Verification items for the finished model (mm, model axes). Coordinates: 2 decimals unless noted, no trailing zeros. Loops run counter-clockwise (first coordinate to the right, second up) from the corner with the lowest first, then second, coordinate; pieces in that order, holes last. Notation, with made-up numbers: (-13.75, 57) - (25.25, 57) arc R17 ccw to (25.25, 69) - close; hole circle Ø2 at (28.25, 78). An arc over 180 degrees is marked (long way). One line per item, written item: value. Start each with the question number.
(1) Section check B-B (z = -86). Count the separate pieces of the cut face and the enclosed holes in it, plus the area to 3 significant figures.
(2) Gauge pin test, flat ends, axial feed: P1, Ø20, axis at x = 83, z = -86, coming from the +Y side; P2, Ø6, axis at x = 338, z = -248, coming from the +Y side. Record the tip position at first contact, or that the pin passes through.
(3) Thickness scan on probe 1 along X at (y, z) = (-26, -86); probe 2 along X at (y, z) = (-2, -86); probe 3 along Z at (x, y) = (570.5, -4). Record the ranges inside material, lowest first. Write a range as [from, to].
(4) Section check A-A (x = 36). Record the boundary of the cut face in (y, z), plus the area to 3 significant figures.
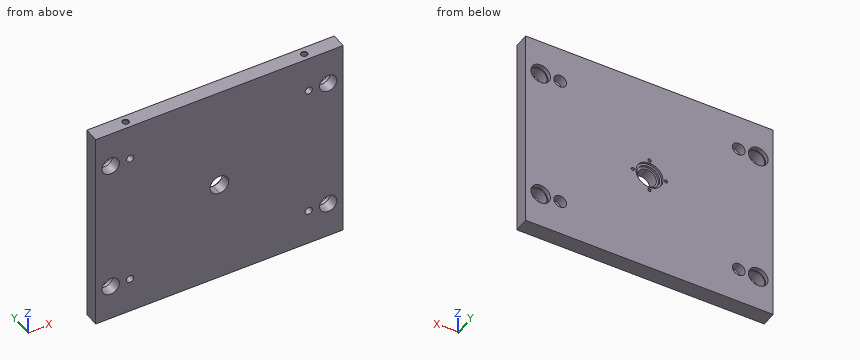
```python
from build123d import *

# Parameters (mm, degrees)
SZKIC1_W                                           = 596
SZKIC1_H                                           = 496
SZKIC1_R                                           = 45
SZKIC1_R_2                                         = 21
DODANIE_WYCI_GNI_CIE1_DEPTH                        = 36
POG_BIENIE_WALCOWE_POD_M16_WKR_T_Z_BEM_D           = 17.5
POG_BIENIE_WALCOWE_POD_M16_WKR_T_Z_BEM_CBORE_D     = 30.713
POG_BIENIE_WALCOWE_POD_M16_WKR_T_Z_BEM_CBORE_DEPTH = 21
SZKIC8_R                                           = 23.5
WYTNIJ_WYCI_GNI_CIE1_DEPTH                         = 10
WYTNIJ_WYCI_GNI_CIE3_DEPTH                         = 777.226770989
WYTNIJ_WYCI_GNI_CIE4_DEPTH                         = 10
WYTNIJ_WYCI_GNI_CIE5_DEPTH                         = 5
OTW_R_GWINTOWANY_M161_D                            = 14
OTW_R_GWINTOWANY_M161_DEPTH                        = 42
OTW_R_GWINTOWANY_M161_CSINK_D                      = 16.05
OTW_R_GWINTOWANY_M161_CSINK_ANGLE                  = 90
OTW_R_GWINTOWANY_M161_TIP                          = 4.206024333
OTW_R_GWINTOWANY_M81_D                             = 6.8
OTW_R_GWINTOWANY_M81_DEPTH                         = 22.25
OTW_R_GWINTOWANY_M81_CSINK_D                       = 8.05
OTW_R_GWINTOWANY_M81_CSINK_ANGLE                   = 90
OTW_R_GWINTOWANY_M81_TIP                           = 2.042926105


with BuildPart() as part:
    # Szkic1 → Dodanie-wyci_gni_cie1 (new body)
    # profile 1 of 2: a face of its own
    with BuildSketch(Plane(origin=(0, 0, 0), x_dir=(1, 0, 0), z_dir=(0, 1, 0))):
        with Locations((298, 248)):
            Rectangle(SZKIC1_W, SZKIC1_H)
        with Locations((298, 248)):
            Circle(SZKIC1_R, mode=Mode.SUBTRACT)
        with Locations(Location((560, 410, 0), (0, 0, 270))):
            Circle(SZKIC1_R_2, mode=Mode.SUBTRACT)
        with Locations(Location((36, 410, 0), (0, 0, 270))):
            Circle(SZKIC1_R_2, mode=Mode.SUBTRACT)
        with Locations(Location((560, 86, 0), (0, 0, 270))):
            Circle(SZKIC1_R_2, mode=Mode.SUBTRACT)
        with Locations(Location((36, 86, 0), (0, 0, 270))):
            Circle(SZKIC1_R_2, mode=Mode.SUBTRACT)
    # profile 2 of 2: a face of its own
    with BuildSketch(Plane(origin=(0, 0, 0), x_dir=(1, 0, 0), z_dir=(0, 1, 0))):
        with Locations((298, 248)):
            Circle(SZKIC1_R)
    extrude(amount=-DODANIE_WYCI_GNI_CIE1_DEPTH)

    # Pog_bienie walcowe pod M16 Wkr_t z _bem (through all)
    with Locations(Plane(origin=(83, 0, -410), x_dir=(0, 0, 1), z_dir=(0, 1, 0))):
        with Locations((0, 0), (0, 430), (324, 430), (324, 0)):
            CounterBoreHole(POG_BIENIE_WALCOWE_POD_M16_WKR_T_Z_BEM_D / 2, POG_BIENIE_WALCOWE_POD_M16_WKR_T_Z_BEM_CBORE_D / 2, POG_BIENIE_WALCOWE_POD_M16_WKR_T_Z_BEM_CBORE_DEPTH)

    # Szkic8 → Wytnij-wyci_gni_cie1 (cut)
    with BuildSketch(Plane(origin=(0, 0, 0), x_dir=(1, 0, 0), z_dir=(0, 1, 0))):
        with Locations(Location((36, 410, 0), (0, 0, 270))):
            Circle(SZKIC8_R)
        with Locations(Location((560, 410, 0), (0, 0, 90))):
            Circle(SZKIC8_R)
        with Locations(Location((560, 86, 0), (0, 0, 270))):
            Circle(SZKIC8_R)
        with Locations(Location((36, 86, 0), (0, 0, 90))):
            Circle(SZKIC8_R)
    extrude(amount=-WYTNIJ_WYCI_GNI_CIE1_DEPTH, mode=Mode.SUBTRACT)

    # Szkic10 → Wytnij-wyci_gni_cie3 (cut, through all)
    with BuildSketch(Plane(origin=(0, 0, 0), x_dir=(1, 0, 0), z_dir=(0, 1, 0))):
        with BuildLine():
            ThreePointArc((320.5, 248), (313.909902577, 263.909902577), (298, 270.5))
            Line((298, 270.5), (298, 225.5))
            ThreePointArc((298, 225.5), (313.909902577, 232.090097423), (320.5, 248))
        make_face()
        with BuildLine():
            Line((298, 225.5), (298, 270.5))
            ThreePointArc((298, 270.5), (275.5, 248), (298, 225.5))
        make_face()
    extrude(amount=-WYTNIJ_WYCI_GNI_CIE3_DEPTH, mode=Mode.SUBTRACT)

    # Szkic10_3 → Wytnij-wyci_gni_cie4 (cut)
    with BuildSketch(Plane(origin=(0, 0, 0), x_dir=(1, 0, 0), z_dir=(0, 1, 0))):
        with BuildLine():
            ThreePointArc((325.5, 248), (317.445436483, 267.445436483), (298, 275.5))
            Line((298, 275.5), (298, 270.5))
            ThreePointArc((298, 270.5), (313.909902577, 263.909902577), (320.5, 248))
            ThreePointArc((320.5, 248), (313.909902577, 232.090097423), (298, 225.5))
            Line((298, 225.5), (298, 220.5))
            ThreePointArc((298, 220.5), (317.445436483, 228.554563517), (325.5, 248))
        make_face()
        with BuildLine():
            Line((298, 270.5), (298, 275.5))
            ThreePointArc((298, 275.5), (270.5, 248), (298, 220.5))
            Line((298, 220.5), (298, 225.5))
            ThreePointArc((298, 225.5), (275.5, 248), (298, 270.5))
        make_face()
    extrude(amount=-WYTNIJ_WYCI_GNI_CIE4_DEPTH, mode=Mode.SUBTRACT)

    # Szkic10_4 → Wytnij-wyci_gni_cie5 (cut)
    with BuildSketch(Plane(origin=(0, 0, 0), x_dir=(1, 0, 0), z_dir=(0, 1, 0))):
        with BuildLine():
            ThreePointArc((330.5, 248), (320.980970389, 270.980970389), (298, 280.5))
            Line((298, 280.5), (298, 275.5))
            ThreePointArc((298, 275.5), (317.445436483, 267.445436483), (325.5, 248))
            ThreePointArc((325.5, 248), (317.445436483, 228.554563517), (298, 220.5))
            Line((298, 220.5), (298, 215.5))
            ThreePointArc((298, 215.5), (320.980970389, 225.019029611), (330.5, 248))
        make_face()
        with BuildLine():
            Line((298, 275.5), (298, 280.5))
            ThreePointArc((298, 280.5), (265.5, 248), (298, 215.5))
            Line((298, 215.5), (298, 220.5))
            ThreePointArc((298, 220.5), (270.5, 248), (298, 275.5))
        make_face()
    extrude(amount=-WYTNIJ_WYCI_GNI_CIE5_DEPTH, mode=Mode.SUBTRACT)

    # Otw_r gwintowany M161
    with Locations(Plane(origin=(513, -18, 0), x_dir=(1, 0, 0), z_dir=(0, 0, 1))):
        with Locations((0, 0), (-430, 0)):
            CounterSinkHole(OTW_R_GWINTOWANY_M161_D / 2, OTW_R_GWINTOWANY_M161_CSINK_D / 2, depth=OTW_R_GWINTOWANY_M161_DEPTH, counter_sink_angle=OTW_R_GWINTOWANY_M161_CSINK_ANGLE)
            with Locations((0, 0, -(OTW_R_GWINTOWANY_M161_DEPTH + OTW_R_GWINTOWANY_M161_TIP / 2))):  # 118° drill point
                Cone(0, OTW_R_GWINTOWANY_M161_D / 2, OTW_R_GWINTOWANY_M161_TIP, mode=Mode.SUBTRACT)

    # Otw_r gwintowany M81
    with Locations(Plane(origin=(258, 0, -248), x_dir=(0, 0, 1), z_dir=(0, 1, 0))):
        with Locations((0, 0), (-40, 40), (0, 80), (40, 40)):
            CounterSinkHole(OTW_R_GWINTOWANY_M81_D / 2, OTW_R_GWINTOWANY_M81_CSINK_D / 2, depth=OTW_R_GWINTOWANY_M81_DEPTH, counter_sink_angle=OTW_R_GWINTOWANY_M81_CSINK_ANGLE)
            with Locations((0, 0, -(OTW_R_GWINTOWANY_M81_DEPTH + OTW_R_GWINTOWANY_M81_TIP / 2))):  # 118° drill point
                Cone(0, OTW_R_GWINTOWANY_M81_D / 2, OTW_R_GWINTOWANY_M81_TIP, mode=Mode.SUBTRACT)


solid = part.part
```
Responses:
1. separate pieces: 5
1. enclosed holes: 0
1. area: 16,500 mm²
2. P1: stops at y = -21
2. P2: stops at y = -22.49
3. probe 1: x = [0, 15], [57, 74.25], [91.75, 504.25], [521.75, 539], [581, 596]
3. probe 2: x = [0, 12.5], [59.5, 67.64], [98.36, 497.64], [528.36, 536.5], [583.5, 596]
3. probe 3: z = [-496, -431.02], [-388.98, -107.02], [-64.98, 0]
4. outline: (-36, -496) - (0, -496) - (0, -433.5) - (-10, -433.5) - (-10, -431) - (-36, -431) - close; (-36, -389) - (-10, -389) - (-10, -386.5) - (0, -386.5) - (0, -109.5) - (-10, -109.5) - (-10, -107) - (-36, -107) - close; (-36, -65) - (-10, -65) - (-10, -62.5) - (0, -62.5) - (0, 0) - (-36, 0) - close
4. area: 14,700 mm²
